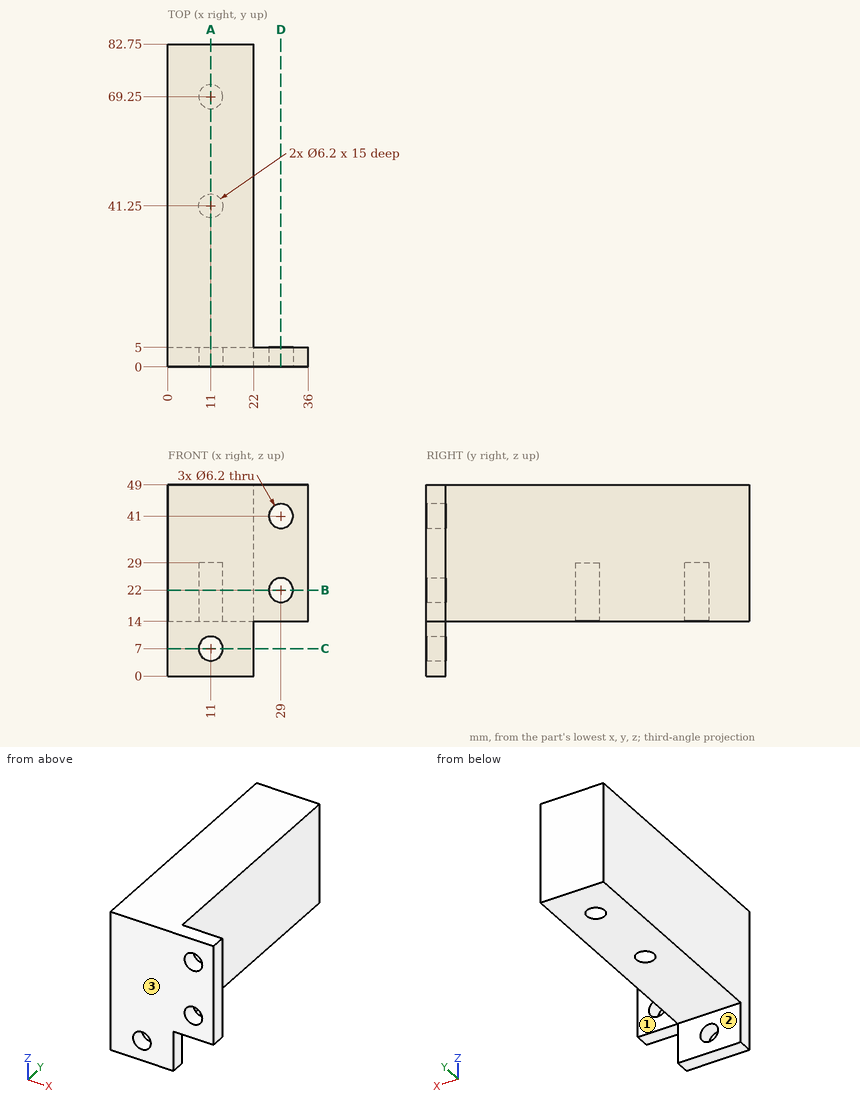
Input: dimensioned drawing with shaded views. Units: mm. Origin: part minimum x, y, z. A direction names the side the tool comes from. Round coordinates to 2 decimals unless told otherwise and drop trailing zeros. Write each loop counter-clockwise with the first axis right and the second up, starting at its lowest first coordinate (ties: lowest second). Pieces come first, ordered by that corner, then holes. Notation, with made-up numbers: (-36, -40) - (11, -40) arc R15 ccw to (11, -29) - close; hole circle Ø8 at (-32, 8.5). An arc over 180 degrees is marked (long way). Write item = value, one per line.
(1) Section query A-A on x = 11. Output: boundary loops of the cut face in (y, z).
Geometry check:
outline = (0, 0) - (5, 0) - (5, 3.9) - (0, 3.9) - close; (0, 10.1) - (5, 10.1) - (5, 14) - (38.15, 14) - (38.15, 29) - (44.35, 29) - (44.35, 14) - (66.15, 14) - (66.15, 29) - (72.35, 29) - (72.35, 14) - (82.75, 14) - (82.75, 49) - (0, 49) - close
(2) Section query C-C on z = 7. Output: boundary loops of the cut face in (x, y), then the cut area to 3 significant figures.
Geometry check:
outline = (0, 0) - (7.9, 0) - (7.9, 5) - (0, 5) - close; (14.1, 0) - (22, 0) - (22, 5) - (14.1, 5) - close
area = 79.0 mm^2
(3) Material intervals for probe 1 along Y at (x, z) = (11, 18); probe 2 along Y at (x, z) = (13.5, 21); probe 3 along X at (y, z) = (1.35, 22), sorted ascending.
Geometry check:
probe_1 = 0 to 38.15, 44.35 to 66.15, 72.35 to 82.75
probe_2 = 0 to 39.42, 43.08 to 67.42, 71.08 to 82.75
probe_3 = 0 to 25.9, 32.1 to 36
(4) Section query B-B on z = 22. Output: boundary loops of the cut face in (x, y), then the cut area to 3 significant figures.
Geometry check:
outline = (0, 0) - (25.9, 0) - (25.9, 5) - (22, 5) - (22, 82.75) - (0, 82.75) - close; (32.1, 0) - (36, 0) - (36, 5) - (32.1, 5) - close; hole circle Ø6.2 at (11, 41.25); hole circle Ø6.2 at (11, 69.25)
area = 1,800 mm^2
(5) Section query D-D on x = 29. Output: boundary loops of the cut face in (y, z), then the cut area to 3 significant figures.
Geometry check:
outline = (0, 14) - (5, 14) - (5, 18.9) - (0, 18.9) - close; (0, 25.1) - (5, 25.1) - (5, 37.9) - (0, 37.9) - close; (0, 44.1) - (5, 44.1) - (5, 49) - (0, 49) - close
area = 113 mm^2
(6) Contact query for flat-ended pins moving along their axis: pin 1 Ø4 at (x, y) = (31, 1.5) entering from -Z; pin 2 Ø3 at (x, y) = (10.5, 69.5) entering from -Z; pin 3 Ø7 at (x, z) = (10.5, 6.5) entering from +Y; pin 4 Ø8 at (x, y) = (27.5, 53) entering from -Z (1 decimal). Output: stop coordinate, or through.
Geometry check:
pin_1 = 14
pin_2 = 29
pin_3 = 5
pin_4 = through
(7) Access query for the marked faces 1, 2 and 3. Directions: +Z, -Z, +X, -X, +Y, -Y. A direction counts if a zero-diameter tool reaches every point of the face in a straight line with its end or side. Return the directions, or none.
Geometry check:
face_1 = +Z, -Z, +X, +Y
face_2 = -Z, +X, -X, +Y
face_3 = +Z, -Z, +X, -X, -Y
